Model file for the job. Use its own axes, mm. Coordinates: 2 decimals unless noted, no trailing zeros. Order: outer loops, then holes, each group sorted by start corner. A loop starts at its lowest first (then second) coordinate and runs counter-clockwise, first axis right, second up. Notation, with made-up numbers: (71.25, 56) -> (128.25, 56) arc R30 ccw to (128.25, 95) -> close; hole circle Ø1 at (-3.75, -4.5). An arc over 180 degrees is marked (long way). Return JSON: item names as keys, results as strings. Group by question number.
1) Pull direction Z, two halves, no side cores. Call faces 1 (the conical face through (-1.513, 2.084, -3.589)), 2 (the cylindrical face through (0.02, 2.05, -0.27)), 3 (the conical face through (-1.51, 2.07, 3.6)), 4 (the conical face through (-1.513, 4.15, 0.01)): +Z half, -Z half, draft (parallel to the pull), parting line (faces both ways), or undercut.
2) Cut at A-A (x = -0.5). Write the cut outline in (y, z).
3) Cut at B-B (x = 1.35). Write the cut outline in (y, z).
4) Probe line 1 (Y direction, x = -1.5, z = -1.5); line 2 (Z direction, x = 1.2, y = 0.5); line 3 (Y direction, x = 0.75, z = -1.75). List the from-to ranges inside material, lowest first.
5) Flat gauge pins, fed straight in: pin 1 (1.5 mm diameter, centred on x = 0, y = -3, fed in from +Z); pin 2 (1 mm diameter, centred on x = 0, z = -2.5, fed in from +Y). Where does each tip first touch, or does it go through?
from build123d import *

# Parameters (mm, degrees)
CUT_EXTRUDE_1_DEPTH      = 3.2
CUT_EXTRUDE_1_DEPTH_BACK = 3.2
SKETCH_2_W               = 18.4
SKETCH_2_H               = 18.4


with BuildPart() as part:
    # Sketch 1 → Revolve 1 (revolve)
    with BuildSketch(Plane.XY, mode=Mode.PRIVATE) as revolve_1_sk:
        Polygon((-1.6, 0), (-1.6, 4), (-1.138119785, 4.8), (1.138119785, 4.8), (1.6, 4), (1.6, 0), align=None)
    revolve(revolve_1_sk.sketch.rotate(Axis((1.6, 0, 0), (-1, 0, 0)), 270), axis=Axis((1.6, 0, 0), (-1, 0, 0)))

    # Sketch 2 → Cut-Extrude 1 (cut, two sides: drawn at the far end of the back side and taken through both)
    with BuildSketch(Plane(origin=(0, 0, 0), x_dir=(0, 0, -1), z_dir=(1, 0, 0)).offset(-CUT_EXTRUDE_1_DEPTH_BACK)):
        Rectangle(SKETCH_2_W, SKETCH_2_H)
        Polygon((-4, 2.309401077), (-4, -2.309401077), (0, -4.618802154), (4, -2.309401077), (4, 2.309401077), (0, 4.618802154), align=None, mode=Mode.SUBTRACT)
    extrude(amount=CUT_EXTRUDE_1_DEPTH + CUT_EXTRUDE_1_DEPTH_BACK, mode=Mode.SUBTRACT)

    # Sketch 3 → Cut-Revolve 1 (revolve, cut)
    with BuildSketch(Plane.XY, mode=Mode.PRIVATE) as cut_revolve_1_sk:
        Polygon((-1.6, 0), (-1.6, 2.5), (-1.167, 2.067), (1.167, 2.067), (1.6, 2.5), (1.6, 0), align=None)
    revolve(cut_revolve_1_sk.sketch.rotate(Axis((1.6, 0, 0), (-1, 0, 0)), 270), axis=Axis((1.6, 0, 0), (-1, 0, 0)), mode=Mode.SUBTRACT)


solid = part.part
Answers below:
{
 "1": {"face 1": "-Z half", "face 2": "undercut", "face 3": "+Z half", "face 4": "parting line"},
 "2": {"outline": "(-4.62, 0) -> (-2.31, -4) -> (2.31, -4) -> (4.62, 0) -> (2.31, 4) -> (-2.31, 4) -> close; hole circle Ø4.13 at (0, 0)"},
 "3": {"outline": "(-4.42, -0.35) -> (-2.51, -3.65) arc R4.43 ccw to (-1.91, -4) -> (1.91, -4) arc R4.43 ccw to (2.51, -3.65) -> (4.42, -0.35) arc R4.43 ccw to (4.42, 0.35) -> (2.51, 3.65) arc R4.43 ccw to (1.91, 4) -> (-1.91, 4) arc R4.43 ccw to (-2.51, 3.65) -> (-4.42, 0.35) arc R4.43 ccw to start; hole circle Ø4.5 at (0, 0)"},
 "4": {"line 1": "y = -3.75 to -1.87, 1.87 to 3.75", "line 2": "z = -4 to -2.04, 2.04 to 4", "line 3": "y = -3.61 to -1.1, 1.1 to 3.61"},
 "5": {"pin 1": "stops at z = 4", "pin 2": "stops at y = 3.46"}
}
